Verification items for the finished model (mm, model axes). Face numbers are marked on the shaded views. A direction names the side the tool comes from. Round coordinates to 2 decimals unless told otherwise and drop trailing zeros. Order: outer loops, then holes, each group sorted by start corner. A loop starts at its lowest first (then second) coordinate and runs counter-clockwise, first axis right, second up.
```python
from build123d import *

# Parameters (mm, degrees)
F1_DEPTH = 88.9


with BuildPart() as f1:
    # F0 (on Top) → F1 (new body)
    with BuildSketch(Plane.XY):
        with BuildLine():
            Line((-35.56, 0), (0, 0))
            Line((0, 0), (35.56, 0))
            ThreePointArc((35.56, 0), (37.570369, 0.987577), (38.017435, 3.182348))
            Line((38.017435, 3.182348), (25.234871, 52.084696))
            ThreePointArc((25.234871, 52.084696), (24.6769, 57.423813), (25.737889, 62.686113))
            Line((25.737889, 62.686113), (30.689125, 76.229293))
            ThreePointArc((30.689125, 76.229293), (29.17569, 79.487009), (25.917974, 77.973574))
            Line((25.917974, 77.973574), (20.966737, 64.430393))
            ThreePointArc((20.966737, 64.430393), (19.602608, 57.664578), (20.32, 50.8))
            Line((20.32, 50.8), (31.438899, 8.262348))
            ThreePointArc((31.438899, 8.262348), (30.991832, 6.067577), (28.981464, 5.08))
            Line((28.981464, 5.08), (0, 5.08))
            Line((0, 5.08), (-28.981464, 5.08))
            ThreePointArc((-28.981464, 5.08), (-30.991832, 6.067577), (-31.438899, 8.262348))
            Line((-31.438899, 8.262348), (-20.32, 50.8))
            ThreePointArc((-20.32, 50.8), (-19.602608, 57.664578), (-20.966737, 64.430393))
            Line((-20.966737, 64.430393), (-25.917974, 77.973574))
            ThreePointArc((-25.917974, 77.973574), (-29.17569, 79.487009), (-30.689125, 76.229293))
            Line((-30.689125, 76.229293), (-25.737889, 62.686113))
            ThreePointArc((-25.737889, 62.686113), (-24.6769, 57.423813), (-25.234871, 52.084696))
            Line((-25.234871, 52.084696), (-38.017435, 3.182348))
            ThreePointArc((-38.017435, 3.182348), (-37.570369, 0.987577), (-35.56, 0))
        make_face()
    extrude(amount=F1_DEPTH)


solid = f1.part
```
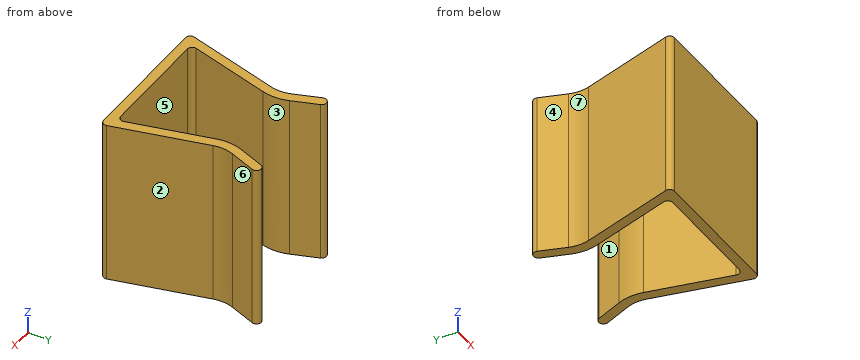
1) Go/stop test with flat-tipped pins: pin 1 Ø6 at (y, z) = (40, 13) entering from -X; pin 2 Ø10 at (y, z) = (23, 28.5) entering from -X; pin 3 Ø8 at (y, z) = (49, 58) entering from -X. Record where each tip stops, or that it passes through.
2) Draft check along X on the marked faces 5, 6 and 7. Enter one of: released by +X, released by -X, zero draft, split by the parting line, or undercut.
3) Sectioned sample at B-B on x = -23. Record the cut outline in (y, z), then the cut area to 3 significant figures.
4) Sectioned sample at D-D on x = 5.5. Record the cut outline in (y, z), then the cut area to 3 significant figures.
5) Tool access check on the marked faces 1, 2, 3 and 4. Record the directions out of +Z, -Z, +X, -X, +Y, -Y that give a thin tool (end or side, any length) a straight path to the whole face; none if there is none.
6) Sectioned sample at C-C on z = 18. Record the cut outline in (x, y), then the cut area to 3 significant figures.
7) Scan lines: probe 1 along Y at (x, z) = (0, 22); probe 2 along X at (y, z) = (64.5, 31); probe 3 along X at (y, z) = (35, 13). Record each from-to range of solid material in increasing order.
8) Sectioned sample at A-A on y = 57.5. Record the cut outline in (x, z).
Returned:
1. pin 1: stops at x = -29.18
1. pin 2: stops at x = -34.14
1. pin 3: stops at x = -27.09
2. face 5: undercut
2. face 6: released by +X
2. face 7: released by -X
3. outline: (0, 0) - (5.08, 0) - (5.08, 88.9) - (0, 88.9) - close; (40.55, 0) - (69.99, 0) - (69.99, 88.9) - (40.55, 88.9) - close
3. area: 3,070 mm2
4. outline: (0, 0) - (5.08, 0) - (5.08, 88.9) - (0, 88.9) - close
4. area: 452 mm2
5. face 1: +Z, -Z, +Y
5. face 2: +Z, -Z, +X
5. face 3: +Z, -Z
5. face 4: +Z, -Z, -X
6. outline: (-38.02, 3.18) arc R2.54 ccw to (-35.56, 0) - (35.56, 0) arc R2.54 ccw to (38.02, 3.18) - (25.23, 52.08) arc R17.78 cw to (25.74, 62.69) - (30.69, 76.23) arc R2.54 ccw to (25.92, 77.97) - (20.97, 64.43) arc R22.86 ccw to (20.32, 50.8) - (31.44, 8.26) arc R2.54 cw to (28.98, 5.08) - (-28.98, 5.08) arc R2.54 cw to (-31.44, 8.26) - (-20.32, 50.8) arc R22.86 ccw to (-20.97, 64.43) - (-25.92, 77.97) arc R2.54 ccw to (-30.69, 76.23) - (-25.74, 62.69) arc R17.78 cw to (-25.23, 52.08) - close
6. area: 1,170 mm2
7. probe 1: y = 0 to 5.08
7. probe 2: x = -26.4 to -20.99, 20.99 to 26.4
7. probe 3: x = -29.7 to -24.45, 24.45 to 29.7
8. outline: (-24.68, 0) - (-19.6, 0) - (-19.6, 88.9) - (-24.68, 88.9) - close; (19.6, 0) - (24.68, 0) - (24.68, 88.9) - (19.6, 88.9) - close
